Geometry: final body of the model. Coordinates: model frame, mm. A direction names the side the tool comes from. Give positions to 0.01 mm unless a question says otherwise; leave off trailing zeros. Loops run counter-clockwise (first coordinate to the right, second up) from the corner with the lowest first, then second, coordinate; pieces in that order, holes last. Notation, with made-up numbers: (-26, -5.5) -> (7, -5.5) arc R32 cw to (7, 24.5) -> close; hole circle Ø2 at (36, 30.5). An arc over 180 degrees is marked (long way). Answer in a Markdown table with one row per item. Add a question column.
1) Section query D-D (y = 7.75). Give the number of separate pieces and of enclosed holes in the cut face, plus the area to 3 significant figures.
2) First-contact query: P1, Ø1.5, axis at y = 4.5, z = -57, coming from the -X side; P2, Ø3, axis at x = 36.25, z = -62.79, coming from the -Y side; P3, Ø4, axis at x = -22, y = 2, coming from the +Z side; P4, Ø1.5, axis at y = 4, z = 20.5, coming from the -X side. Flat tips, straight axial feed; report the tip coordinate or a pass-through.
3) Section query C-C (z = -32.5). Return the cut outline in (x, y).
4) Section query B-B (z = 0). Return the cut outline in (x, y).
5) Line query: line 1 (Z direction, x = 72.5, y = 5.75); line 2 (Z direction, x = -36.25, y = 4); line 3 (Z direction, x = 47, y = 4.25). Output: solid intervals per line, ascending. Write a range as from..to.
6) Access query for faces 1 (the flat face through (-66, 10, 0)), 2 (the cylindrical face through (-56, 5, -33)). Directions: +Z, -Z, +X, -X, +Y, -Y. A direction counts if a zero-diameter tool reaches every point of the face in a straight line with its end or side. Return the directions, or none.
7) Section query A-A (x = 0). Return the cut outline in (y, z), plus the area to 3 significant figures.
8) Draft query along Z for faces 3 (the cylindrical face through (-3.517, 5.07, 79.923)), 4 (the flat face through (-66, 0, 0)), 5 (the flat face through (62.447, 5.07, 28.703)). Return one class per face: +Z half, -Z half, draft (parallel to the pull), parting line (faces both ways), or undercut.
```python
from build123d import *

# Parameters (mm, degrees)
SKETCH2_W                    = 15
SKETCH2_H                    = 10
CUT_EXTRUDE1_DEPTH           = 114.578166916
FILLET1_R                    = 1.5
CIRPATTERN2_COUNT            = 3
FILLET1_OF_CIRPATTERN2_R     = 1.5
F_10_0_1935_DIAMETER_HOLE1_D = 4.9149
CIRPATTERN3_COUNT            = 6


with BuildPart() as part:
    # Sketch2 → Revolve1 (revolve)
    with BuildSketch(Plane(origin=(0, 0, 0), x_dir=(0, 0, -1), z_dir=(1, 0, 0)), mode=Mode.PRIVATE) as revolve1_sk:
        with Locations((-72.5, 5)):
            Rectangle(SKETCH2_W, SKETCH2_H)
    revolve(revolve1_sk.sketch.rotate(Axis((0, -0.75, 0), (0, 1, 0)), 180), axis=Axis((0, -0.75, 0), (0, 1, 0)))

    # Sketch4 → Cut-Extrude1 (cut, through all)
    with BuildSketch(Plane(origin=(0, 10, 0), x_dir=(1, 0, 0), z_dir=(0, 1, 0))):
        with BuildLine():
            Line((-3.881158746, 64.88402428), (-8.835527397, 71.959595994))
            ThreePointArc((-8.835527397, 71.959595994), (0, 72.5), (8.835527397, 71.959595994))
            Line((8.835527397, 71.959595994), (3.881158746, 64.88402428))
            ThreePointArc((3.881158746, 64.88402428), (0, 65), (-3.881158746, 64.88402428))
        make_face()
    cut_extrude1 = extrude(amount=-CUT_EXTRUDE1_DEPTH, mode=Mode.SUBTRACT)

    # Fillet1
    fillet1_edges = [part.edges().sort_by_distance(p)[0] for p in [
        (3.881158746, 5, -64.88402428),
        (-3.881158746, 5, -64.88402428),
        (-8.835527397, 5, -71.959595994),
        (8.835527397, 5, -71.959595994),
    ]]
    fillet(fillet1_edges, radius=FILLET1_R)

    # CirPattern2: Cut-Extrude1 ×3 about axis
    cirpattern2_axis = Axis((0, 0, 0), (0, 1, 0))
    for i in range(1, CIRPATTERN2_COUNT):
        add(cut_extrude1.rotate(cirpattern2_axis, i * 360 / CIRPATTERN2_COUNT), mode=Mode.SUBTRACT)

    # Fillet1 of CirPattern2
    fillet1_of_cirpattern2_edges = [part.edges().sort_by_distance(p)[0] for p in [
        (-58.131792699, 5, 29.08083007),
        (-54.250633954, 5, 35.80319421),
        (-57.901074478, 5, 43.631589179),
        (-66.736601875, 5, 28.328006815),
        (54.250633954, 5, 35.80319421),
        (58.131792699, 5, 29.08083007),
        (66.736601875, 5, 28.328006815),
        (57.901074478, 5, 43.631589179),
    ]]
    fillet(fillet1_of_cirpattern2_edges, radius=FILLET1_OF_CIRPATTERN2_R)

    # #10 (0.1935) Diameter Hole1 (through all)
    with Locations(Plane(origin=(0, 10, 0), x_dir=(1, 0, 0), z_dir=(0, 1, 0))):
        with Locations((-36.25, 62.786841774)):
            f_10_0_1935_diameter_hole1 = Hole(F_10_0_1935_DIAMETER_HOLE1_D / 2)

    # CirPattern3: #10 (0.1935) Diameter Hole1 ×6 about axis
    cirpattern3_axis = Axis((0, 0, 0), (0, 1, 0))
    for i in range(1, CIRPATTERN3_COUNT):
        add(f_10_0_1935_diameter_hole1.rotate(cirpattern3_axis, i * 360 / CIRPATTERN3_COUNT), mode=Mode.SUBTRACT)


solid = part.part
```
Evaluation:
| question | item | result |
|---|---|---|
| 1 | separate pieces | 1 |
| 1 | enclosed holes | 7 |
| 1 | area | 6,430 mm² |
| 2 | P1 | x = -56.89 |
| 2 | P2 | through |
| 2 | P3 | z = 77.46 |
| 2 | P4 | x = -77.52 |
| 3 | outline | (-73.1, 0) -> (-56.29, 0) -> (-56.29, 10) -> (-73.1, 10) -> close; (56.29, 0) -> (73.1, 0) -> (73.1, 10) -> (56.29, 10) -> close |
| 4 | outline | (-80, 0) -> (-74.96, 0) -> (-74.96, 10) -> (-80, 10) -> close; (-70.04, 0) -> (-65, 0) -> (-65, 10) -> (-70.04, 10) -> close; (65, 0) -> (70.04, 0) -> (70.04, 10) -> (65, 10) -> close; (74.96, 0) -> (80, 0) -> (80, 10) -> (74.96, 10) -> close |
| 5 | line 1 | -33.82..-2.46, 2.46..33.82 |
| 5 | line 2 | -71.32..-65.24, -60.33..-53.95, 53.95..60.33, 65.24..71.32 |
| 5 | line 3 | -64.74..-44.9, 44.9..64.74 |
| 6 | face 1 | +Z, -Z, +X, -X, +Y |
| 6 | face 2 | +Y, -Y |
| 7 | outline | (0, -80) -> (10, -80) -> (10, -72.5) -> (0, -72.5) -> close; (0, 65) -> (10, 65) -> (10, 80) -> (0, 80) -> close |
| 7 | area | 225 mm² |
| 8 | face 3 | parting line |
| 8 | face 4 | draft |
| 8 | face 5 | undercut |
